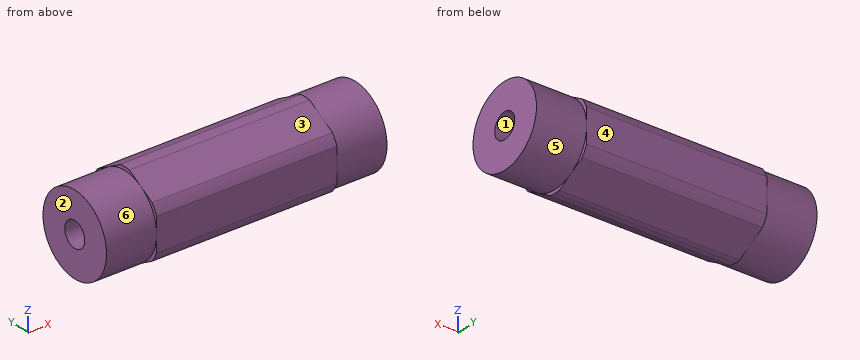
from build123d import *

# Parameters (mm, degrees)
SKETCH1_R               = 2.000000064
BOSS_EXTRUDE1_DEPTH     = 22.225
SKETCH4_R               = 8.89
SKETCH4_R_2             = 6.35
CUT_EXTRUDE_THIN1_DEPTH = 7.9375


with BuildPart() as part:
    # Sketch1 → Boss-Extrude1 (new, symmetric)
    with BuildSketch(Plane(origin=(0, 0, 0), x_dir=(0, 0, -1), z_dir=(1, 0, 0))):
        with BuildLine():
            ThreePointArc((6.874999966, 0), (6.860422465, 0.447468582), (6.816751782, 0.893039571))
            Line((6.816751782, 0.893039571), (4.181770846, 5.456960429))
            ThreePointArc((4.181770846, 5.456960429), (3.437499983, 5.953924622), (2.634980936, 6.35))
            Line((2.634980936, 6.35), (-2.634980936, 6.35))
            ThreePointArc((-2.634980936, 6.35), (-3.437499983, 5.953924622), (-4.181770846, 5.456960429))
            Line((-4.181770846, 5.456960429), (-6.816751782, 0.893039571))
            ThreePointArc((-6.816751782, 0.893039571), (-6.874999966, 0), (-6.816751782, -0.893039571))
            Line((-6.816751782, -0.893039571), (-4.181770846, -5.456960429))
            ThreePointArc((-4.181770846, -5.456960429), (-3.437499983, -5.953924622), (-2.634980936, -6.35))
            Line((-2.634980936, -6.35), (2.634980936, -6.35))
            ThreePointArc((2.634980936, -6.35), (3.437499983, -5.953924622), (4.181770846, -5.456960429))
            Line((4.181770846, -5.456960429), (6.816751782, -0.893039571))
            ThreePointArc((6.816751782, -0.893039571), (6.860422465, -0.447468582), (6.874999966, 0))
        make_face()
        Circle(SKETCH1_R, mode=Mode.SUBTRACT)
    extrude(amount=BOSS_EXTRUDE1_DEPTH, both=True)

    # Sketch4 → Cut-Extrude-Thin1 (cut)
    with BuildSketch(Plane.ZY.offset(22.225)):
        Circle(SKETCH4_R)
        Circle(SKETCH4_R_2, mode=Mode.SUBTRACT)
    cut_extrude_thin1 = extrude(amount=-CUT_EXTRUDE_THIN1_DEPTH, mode=Mode.SUBTRACT)

    # Mirror1: Cut-Extrude-Thin1 across plane
    add(cut_extrude_thin1.mirror(Plane.ZY), mode=Mode.SUBTRACT)


solid = part.part
Verification items for the finished model (mm, model axes). Face numbers are marked on the shaded views. A direction names the side the tool comes from. Coordinates: 2 decimals unless noted, no trailing zeros. Order: outer loops, then holes, each group sorted by start corner. A loop starts at its lowest first (then second) coordinate and runs counter-clockwise, first axis right, second up. Notation, with made-up numbers: (29, 9) -> (57, 9) arc R9 ccw to (57, 21) -> close; hole circle Ø3 at (23.5, -31.5). An arc over 180 degrees is marked (long way). Use CSV: the item, a comma, the result in double quotes. Start each with the question number.
Q1. Section check B-B, the plane y = 0.5. Record the cut outline in (x, z) (1 decimal).
Q2. Section check A-A, the plane x = -13. Record the cut outline in (y, z) (3 decimals).
Q3. Draft check along Y on the marked faces 1, 2 and 3. Enter one of: +Y half, -Y half, draft (parallel to the pull), parting line (faces both ways), or undercut.
Q4. Thickness scan on line 1 along Z through (x, y) = (7, 3.25); line 2 along Z through (x, y) = (-17, 1); line 3 along Z through (x, y) = (2.5, -1) (3 decimals). Record the ranges inside material, lowest first.
Q5. Section check C-C, the plane z = 3.25. Record the cut outline in (x, y) (1 decimal).
Q6. Depth check by flat-ended pin: P1, Ø1, axis at x = 9.5, y = -3.5, coming from the +Z side; P2, Ø1.5, axis at x = -16, y = 3, coming from the -Z side. Enter the tip coordinate at first touch or a pass-through.
Q7. Tool access check on the marked faces 4, 5 and 6. Record the directions out of +Z, -Z, +X, -X, +Y, -Y that give a thin tool (end or side, any length) a straight path to the whole face; none if there is none.
Returned:
1,outline,"(-22.2, -6.3) -> (-14.3, -6.3) -> (-14.3, -6.9) -> (14.3, -6.9) -> (14.3, -6.3) -> (22.2, -6.3) -> (22.2, -1.9) -> (-22.2, -1.9) -> close; (-22.2, 1.9) -> (22.2, 1.9) -> (22.2, 6.3) -> (14.3, 6.3) -> (14.3, 6.9) -> (-14.3, 6.9) -> (-14.3, 6.3) -> (-22.2, 6.3) -> close"
2,outline,"(-6.35, -2.635) arc R6.875 ccw to (-5.457, -4.182) -> (-0.893, -6.817) arc R6.875 ccw to (0.893, -6.817) -> (5.457, -4.182) arc R6.875 ccw to (6.35, -2.635) -> (6.35, 2.635) arc R6.875 ccw to (5.457, 4.182) -> (0.893, 6.817) arc R6.875 ccw to (-0.893, 6.817) -> (-5.457, 4.182) arc R6.875 ccw to (-6.35, 2.635) -> close; hole circle Ø4 at (0, 0)"
3,face 1,"undercut"
3,face 2,"draft"
3,face 3,"-Y half"
4,line 1,"z = -5.46 to 5.46"
4,line 2,"z = -6.27 to -1.73, 1.73 to 6.27"
4,line 3,"z = -6.755 to -1.732, 1.732 to 6.755"
5,outline,"(-22.2, -5.5) -> (-14.3, -5.5) -> (-14.3, -6.1) -> (14.3, -6.1) -> (14.3, -5.5) -> (22.2, -5.5) -> (22.2, 5.5) -> (14.3, 5.5) -> (14.3, 6.1) -> (-14.3, 6.1) -> (-14.3, 5.5) -> (-22.2, 5.5) -> close"
6,P1,"stops at z = 5.6"
6,P2,"stops at z = -5.94"
7,face 4,"+Z, -Z, +X, -X, +Y"
7,face 5,"+X"
7,face 6,"-X"
